Build history of the part. All positions in model axes, mm. Face numbers are marked on the shaded views. A direction names the side the tool comes from. Give positions to 0.01 mm unless a question says otherwise; leave off trailing zeros. Order: outer loops, then holes, each group sorted by start corner. A loop starts at its lowest first (then second) coordinate and runs counter-clockwise, first axis right, second up. Notation, with made-up numbers: (38, 81) - (83, 81) arc R30 cw to (83, 113) - close; hole circle Ø4 at (77.25, 6.25). An arc over 180 degrees is marked (long way). Write each question's results on one line, items separated by ' | '. Start each with the question number.
1) Cut at B-B on x = -13.5. List the corners of the cut face in (y, z).
2) Cut at D-D on x = -26.5. List the corners of the cut face in (y, z), plus the area to 4 significant figures.
3) Drill centre lines: line 1 along X through (y, z) = (18, 8.5); line 2 along Y through (x, z) = (-25, 4.5); line 3 along Y through (x, z) = (-4, 19.5). Where is each one in solid material? Low to high. Write a range as from..to.
4) Cut at A-A on z = 15. List the corners of the cut face in (x, y), plus the area to 3 significant figures.
5) Drop flat-ended pins along their axis: pin 1 Ø4 at (y, z) = (19, 19.5) entering from -X; pin 2 Ø4 at (x, z) = (-13, 7) entering from +Y; pin 3 Ø6 at (x, z) = (-14, 7.5) entering from +Y. Give the stop position or say it passes through.
6) Cut at C-C on y = 6.5. List the corners of the cut face in (x, z), plus the area to 4 significant figures.
7) Tool access for the marked faces 1 and 2: list every direction of +Z, -Z, +X, -X, +Y, -Y with a clear straight run to the whole face (end or side of a thin tool).
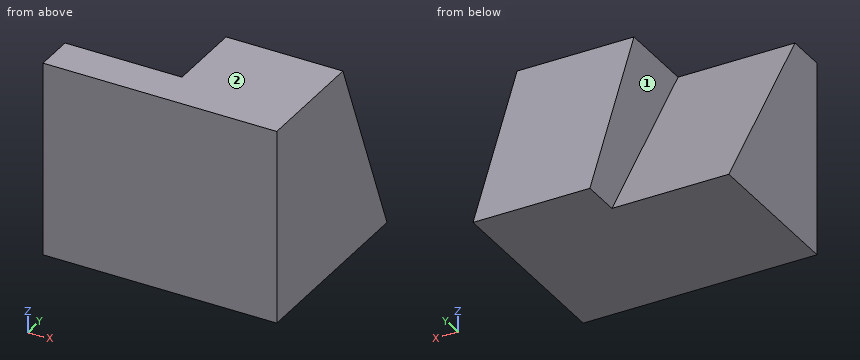
from build123d import *

# Parameters (mm, degrees)
BOSS_EXTRUDE1_DEPTH = 25
BOSS_EXTRUDE2_DEPTH = 15
BOSS_EXTRUDE3_DEPTH = 15


with BuildPart() as part:
    # Sketch1 → Boss-Extrude1 (new body)
    with BuildSketch(Plane.XY):
        Polygon((-30, 5), (-15, 5), (-15, 15), (0, 15), (0, 0), (-30, 0), align=None)
    extrude(amount=BOSS_EXTRUDE1_DEPTH)

    # Sketch2 → Boss-Extrude2 (add)
    with BuildSketch(Plane(origin=(0, 0, 0), x_dir=(0, 0, -1), z_dir=(1, 0, 0))):
        Polygon((0, 15), (0, 25), (-25, 15), align=None)
    extrude(amount=-BOSS_EXTRUDE2_DEPTH)

    # Sketch3 → Boss-Extrude3 (add)
    with BuildSketch(Plane.ZY.offset(15)):
        Polygon((0, 5), (0, 20), (25, 5), align=None)
    extrude(amount=BOSS_EXTRUDE3_DEPTH)


solid = part.part
Results:
1) outline: (0, 0) - (25, 0) - (15, 25) - (0, 25) - close
2) outline: (0, 0) - (20, 0) - (5, 25) - (0, 25) - close | area: 312.5 mm^2
3) line 1: -15..0 | line 2: 0..17.3 | line 3: 0..17.2
4) outline: (-30, 0) - (0, 0) - (0, 19) - (-15, 19) - (-15, 11) - (-30, 11) - close | area: 450 mm^2
5) pin 1: x = -15 | pin 2: y = 23 | pin 3: y = 23.2
6) outline: (-30, 0) - (0, 0) - (0, 25) - (-15, 25) - (-15, 22.5) - (-30, 22.5) - close | area: 712.5 mm^2
7) face 1: +Z, -X, +Y | face 2: +Z, +X, -X, +Y, -Y
